Autodesk Inventor part; units mm, degrees
ref_plane "YZ Plane" through (0, 0, 0) normal (1, 0, 0) x (0, 1, 0)
ref_plane "XZ Plane" through (0, 0, 0) normal (0, 1, 0) x (-1, 0, 0)
ref_plane "XY Plane" through (0, 0, 0) normal (0, 0, 1) x (1, 0, 0)
sketch "Sketch1" plane through (0, 0, 0) normal (0, 0, 1) x (1, 0, 0)
  line L0 (-9.525, 292.1) -> (9.525, 292.1)
  line L1 (9.525, 292.1) -> (9.525, -292.1)
  line L2 (9.525, -292.1) -> (-9.525, -292.1)
  line L3 (-9.525, -292.1) -> (-9.525, 292.1)
  point P0 (0, 0)
  point P1 (9.525, 0)
  point P2 (0, 292.1)
  dimension "d0" = 19.05
  dimension "d1" = 584.2
extrude "Extrusion1" add sketch "Sketch1" along normal blind 3
sketch "Sketch2" plane through (0, 0, 3) normal (0, 0, 1) x (1, 0, 0)
  line L0 (-9.525, 292.1) -> (9.525, 292.1)
  line L1 (9.525, -292.1) -> (-9.525, -292.1)
  point P0 (0, 0)
  point P1 (0, 266.7)
  point P2 (0, 133.35)
  point P3 (0, 0)
  point P4 (0, -133.35)
  point P5 (0, -266.7)
  dimension "d4" = 25.4
  dimension "d5" = 133.35
  dimension "d6" = 133.35
  dimension "d7" = 133.35
  dimension "d8" = 133.35
  dimension "d9" = 25.4
hole "Hole1" at (0, 266.7, 3) at (0, 133.35, 3) at (0, 0, 3) at (0, -133.35, 3) at (0, -266.7, 3) direction (0, 0, -1) diameter 6.35 end through all
properties part number "top panel"
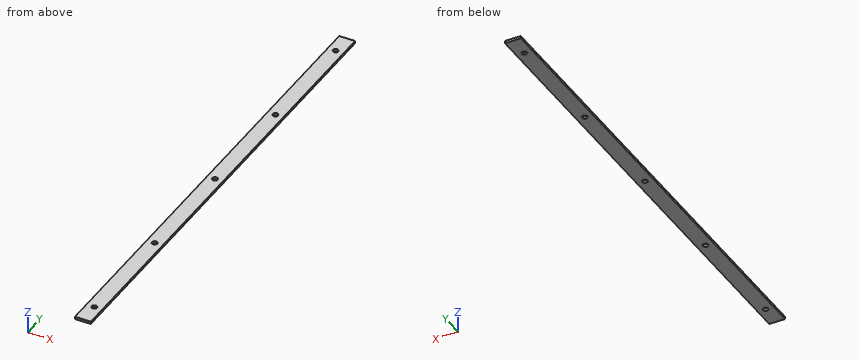
Here's how the part is built. I have some questions about the finished solid (model axes, mm). Coordinates: 2 decimals unless noted, no trailing zeros. Order: outer loops, then holes, each group sorted by start corner. A loop starts at its lowest first (then second) coordinate and runs counter-clockwise, first axis right, second up. Notation, with made-up numbers: M -36.75,14.25 L 11.25,14.25 A15 cw 11.25,26.25 Z; hole C -37.75,16.25 d1. An arc over 180 degrees is marked long. Answer as CSV lines item,"result".
Item 1: Imagine slicing it at A-A on x = 0. Write out the boundary of the cut face in (y, z) (3 decimals), plus the area to 3 significant figures.
Results found:
outline,"M -292.1,0 L -269.875,0 L -269.875,3 L -292.1,3 Z; M -263.525,0 L -136.525,0 L -136.525,3 L -263.525,3 Z; M -130.175,0 L -3.175,0 L -3.175,3 L -130.175,3 Z; M 3.175,0 L 130.175,0 L 130.175,3 L 3.175,3 Z; M 136.525,0 L 263.525,0 L 263.525,3 L 136.525,3 Z; M 269.875,0 L 292.1,0 L 292.1,3 L 269.875,3 Z"
area,"1,660 mm2"
Item 2: For pin 1 (8.5 mm diameter, centred on x = 0, y = -133.35, fed in from +Z), with a flat end and sliding along its axis, tell me the tip position at first contact or that it passes through.
Results found:
pin 1,"z = 3"
Item 3: If I drill on line 1 (Y direction, x = -0.25, z = 2.9); line 2 (X direction, y = 0, z = 1.65) (3 decimals); line 3 (Y direction, x = -2.5, z = 2.45), over which ranges is the centre line in solid material (lowest first)?
Results found:
line 1,"-292.1 to -269.87, -263.53 to -136.52, -130.18 to -3.17, 3.17 to 130.18, 136.52 to 263.53, 269.87 to 292.1"
line 2,"-9.525 to -3.175, 3.175 to 9.525"
line 3,"-292.1 to -268.66, -264.74 to -135.31, -131.39 to -1.96, 1.96 to 131.39, 135.31 to 264.74, 268.66 to 292.1"
